For this review, take the finished solid that the model builds, in its own axes (mm). A direction names the side the tool comes from. Round coordinates to 2 decimals unless told otherwise and drop trailing zeros. Loops run counter-clockwise (first coordinate to the right, second up) from the corner with the lowest first, then second, coordinate; pieces in that order, holes last. Notation, with made-up numbers: (57.5, -3) -> (66.5, -3) arc R18 ccw to (66.5, 31) -> close; hole circle Ø5 at (12.25, 58). An arc over 180 degrees is marked (long way). Use one line per item in the form item = value. Start each with the question number.
from build123d import *

# Parameters (mm, degrees)
BOSS_EXTRUDE1_DEPTH  = 114.3
SKETCH2_W            = 6.35
SKETCH2_H            = 17.78
CUT_EXTRUDE2_DEPTH   = 99.06
SKETCH3_W            = 27.183356596
SKETCH3_H            = 83.82
CUT_EXTRUDE3_DEPTH   = 99.06
SKETCH4_W            = 27.183356596
SKETCH4_H            = 83.82
CUT_EXTRUDE4_DEPTH   = 99.06
SKETCH7_W            = 3.263536018
SKETCH7_H            = 7.713600016
CUT_EXTRUDE7_DEPTH   = 15.24
CUT_EXTRUDE8_DEPTH   = 99.06
SKETCH10_W           = 39.883356596
SKETCH10_H           = 114.3
BOSS_EXTRUDE2_DEPTH  = 7.62
CUT_EXTRUDE11_DEPTH  = 81.28
BOSS_EXTRUDE9_DEPTH  = 4.826
MIRROR9_COPY_1_DEPTH = 4.826
CUT_EXTRUDE13_DEPTH  = 19.941678176
CUT_EXTRUDE14_DEPTH  = 19.941678176
SKETCH17_W           = 27.183356538
SKETCH17_H           = 4.826
CUT_EXTRUDE15_DEPTH  = 99.06
SKETCH18_W           = 39.883356596
SKETCH18_H           = 7.62
CUT_EXTRUDE16_DEPTH  = 19.941678176
SKETCH20_W           = 27.183356538
SKETCH20_H           = 2.54
CUT_EXTRUDE19_DEPTH  = 79.118321824
FILLET1_R            = 5.08
FILLET2_R            = 2.54
SKETCH21_R           = 2.749999961
CUT_EXTRUDE20_DEPTH  = 79.118321824
SKETCH22_W           = 39.883356596
SKETCH22_H           = 5.08
BOSS_EXTRUDE10_DEPTH = 38.1
CUT_EXTRUDE21_REACH  = 169.333


with BuildPart() as part:
    # Sketch1 → Boss-Extrude1 (new body)
    with BuildSketch(Plane(origin=(0, 0, 0), x_dir=(1, 0, 0), z_dir=(0, 1, 0))):
        with BuildLine():
            Line((39.883356596, 0), (19.941678298, 34.54))
            Line((19.941678298, 34.54), (9.525, 34.54))
            Line((9.525, 34.54), (9.525, 52.32))
            Line((9.525, 52.32), (3.175, 52.32))
            Line((3.175, 52.32), (3.175, 34.54))
            Line((3.175, 34.54), (3.175, 29.28841025))
            ThreePointArc((3.175, 29.28841025), (0, -29.46), (-3.175, 29.28841025))
            Line((-3.175, 29.28841025), (-3.175, 34.54))
            Line((-3.175, 34.54), (-3.175, 52.32))
            Line((-3.175, 52.32), (-9.525, 52.32))
            Line((-9.525, 52.32), (-9.525, 34.54))
            Line((-9.525, 34.54), (-19.941678298, 34.54))
            Line((-19.941678298, 34.54), (-39.883356596, 0))
            Line((-39.883356596, 0), (-19.941678298, -34.54))
            Line((-19.941678298, -34.54), (19.941678298, -34.54))
            Line((19.941678298, -34.54), (39.883356596, 0))
        make_face()
    extrude(amount=BOSS_EXTRUDE1_DEPTH)

    # Sketch2 → Cut-Extrude2 (cut)
    with BuildSketch(Plane(origin=(0, 114.3, 0), x_dir=(1, 0, 0), z_dir=(0, 1, 0))):
        with Locations((-6.35, 43.43)):
            Rectangle(SKETCH2_W, SKETCH2_H)
        with Locations((6.35, 43.43)):
            Rectangle(SKETCH2_W, SKETCH2_H)
    extrude(amount=-CUT_EXTRUDE2_DEPTH, mode=Mode.SUBTRACT)

    # Sketch3 → Cut-Extrude3 (cut)
    with BuildSketch(Plane(origin=(-29.912517447, 0, -17.27), x_dir=(-0.49999999999999617, 0, 0.8660254037844409), z_dir=(-0.8660254037844408, 0, -0.4999999999999961))):
        with Locations((0, 57.15)):
            Rectangle(SKETCH3_W, SKETCH3_H)
    extrude(amount=-CUT_EXTRUDE3_DEPTH, mode=Mode.SUBTRACT)

    # Sketch4 → Cut-Extrude4 (cut)
    with BuildSketch(Plane(origin=(29.912517447, 0, -17.27), x_dir=(-0.500000000000004, 0, -0.8660254037844364), z_dir=(0.8660254037844365, 0, -0.500000000000004))):
        with Locations((0, 57.15)):
            Rectangle(SKETCH4_W, SKETCH4_H)
    extrude(amount=-CUT_EXTRUDE4_DEPTH, mode=Mode.SUBTRACT)

    # Sketch7 → Cut-Extrude7 (cut)
    with BuildSketch(Plane.XZ):
        with Locations((-30.838217531, 0)):
            Rectangle(SKETCH7_W, SKETCH7_H)
        with Locations((30.838217531, 0)):
            Rectangle(SKETCH7_W, SKETCH7_H)
    extrude(amount=-CUT_EXTRUDE7_DEPTH, mode=Mode.SUBTRACT)

    # Sketch8 → Cut-Extrude8 (cut)
    with BuildSketch(Plane(origin=(0, 114.3, 0), x_dir=(1, 0, 0), z_dir=(0, 1, 0))):
        Polygon((-3.175, 29.714), (3.175, 29.714), (17.155385899, 29.714), (34.310771797, 0), (17.155385899, -29.714), (-17.155385899, -29.714), (-34.310771797, 0), (-17.155385899, 29.714), align=None)
    extrude(amount=-CUT_EXTRUDE8_DEPTH, mode=Mode.SUBTRACT)

    # Sketch10 → Boss-Extrude2 (add)
    with BuildSketch(Plane.XY.offset(34.54)):
        with Locations((0, 57.15)):
            Rectangle(SKETCH10_W, SKETCH10_H)
    extrude(amount=BOSS_EXTRUDE2_DEPTH)

    # Sketch12 → Cut-Extrude11 (cut)
    with BuildSketch(Plane(origin=(-29.912517447, 0, -17.27), x_dir=(-0.4999999999999998, 0, 0.8660254037844388), z_dir=(-0.8660254037844388, 0, -0.4999999999999998))):
        Polygon((19.941678298, 114.3), (0, 114.3), (19.941678298, 94.358321702), align=None)
        Polygon((-19.941678298, 94.358321702), (0, 114.3), (-19.941678298, 114.3), align=None)
        Polygon((6.259743879, 99.06), (0, 105.319743879), (-6.259743879, 99.06), align=None)
    cut_extrude11 = extrude(amount=-CUT_EXTRUDE11_DEPTH, mode=Mode.SUBTRACT)

    # Mirror2: Cut-Extrude11 across plane
    add(cut_extrude11.mirror(Plane(origin=(0, 0, 0), x_dir=(0, 0, 1), z_dir=(1, 0, 0))), mode=Mode.SUBTRACT)

    # Sketch11 → Boss-Extrude9 (add)
    with BuildSketch(Plane(origin=(-29.912517447, 0, -17.27), x_dir=(-0.4999999999999998, 0, 0.8660254037844388), z_dir=(-0.8660254037844388, 0, -0.4999999999999998))):
        Polygon((-13.591678298, 91.728065581), (0, 105.319743879), (13.591678298, 91.728065581), (19.941678298, 94.358321702), (0, 114.3), (-19.941678298, 94.358321702), align=None)
    boss_extrude9 = extrude(amount=-BOSS_EXTRUDE9_DEPTH)

    # Mirror8: Boss-Extrude9 across plane
    add(boss_extrude9.mirror(Plane.XY))

    # Mirror9: Boss-Extrude9 across plane
    add(boss_extrude9.mirror(Plane(origin=(0, 0, 0), x_dir=(0, 0, 1), z_dir=(1, 0, 0))))

    # Mirror9 copy 1 sketch → Mirror9 copy 1 (add)
    with BuildSketch(Plane(origin=(29.912517447, 0, 17.27), x_dir=(0.4999999999999998, 0, -0.8660254037844388), z_dir=(0.8660254037844388, 0, 0.4999999999999998))):
        Polygon((-13.591678298, 91.728065581), (0, 105.319743879), (13.591678298, 91.728065581), (19.941678298, 94.358321702), (0, 114.3), (-19.941678298, 94.358321702), align=None)
    extrude(amount=-MIRROR9_COPY_1_DEPTH)

    # Sketch15 → Cut-Extrude13 (cut)
    with BuildSketch(Plane(origin=(0, 114.3, 0), x_dir=(1, 0, 0), z_dir=(0, 1, 0))):
        Polygon((-17.155385899, 29.714), (-19.941678298, 34.54), (19.941678298, 34.54), (17.155385899, 29.714), align=None)
    extrude(amount=-CUT_EXTRUDE13_DEPTH, mode=Mode.SUBTRACT)

    # Sketch16 → Cut-Extrude14 (cut)
    with BuildSketch(Plane(origin=(0, 114.3, 0), x_dir=(1, 0, 0), z_dir=(0, 1, 0))):
        Polygon((-19.941678298, -34.54), (19.941678298, -34.54), (11.5828011, -29.714), (-11.5828011, -29.714), align=None)
    extrude(amount=-CUT_EXTRUDE14_DEPTH, mode=Mode.SUBTRACT)

    # Sketch17 → Cut-Extrude15 (cut)
    with BuildSketch(Plane(origin=(0, 114.3, 0), x_dir=(1, 0, 0), z_dir=(0, 1, 0))):
        with Locations((0, -32.127)):
            Rectangle(SKETCH17_W, SKETCH17_H)
    extrude(amount=-CUT_EXTRUDE15_DEPTH, mode=Mode.SUBTRACT)

    # Sketch18 → Cut-Extrude16 (cut)
    with BuildSketch(Plane(origin=(0, 114.3, 0), x_dir=(1, 0, 0), z_dir=(0, 1, 0))):
        with Locations((0, -38.35)):
            Rectangle(SKETCH18_W, SKETCH18_H)
    extrude(amount=-CUT_EXTRUDE16_DEPTH, mode=Mode.SUBTRACT)

    # Sketch20 → Cut-Extrude19 (cut)
    with BuildSketch(Plane(origin=(0, 94.358321824, 0), x_dir=(1, 0, 0), z_dir=(0, 1, 0))):
        with Locations((0, -35.81)):
            Rectangle(SKETCH20_W, SKETCH20_H)
    extrude(amount=-CUT_EXTRUDE19_DEPTH, mode=Mode.SUBTRACT)

    # Fillet1
    fillet1_edges = [part.edges().sort_by_distance(p)[0] for p in [
        (19.941678298, 47.179160851, 34.54),
        (-39.883356596, 47.179160851, 0),
        (-19.941678298, 47.179160851, -34.54),
        (39.883356596, 47.179160851, 0),
        (-19.941678298, 47.179160851, 34.54),
        (19.941678298, 47.179160851, -34.54),
        (-9.525, 7.62, -34.54),
        (9.525, 7.62, -34.54),
    ]]
    fillet(fillet1_edges, radius=FILLET1_R)

    # Fillet2
    fillet2_edges = [part.edges().sort_by_distance(p)[0] for p in [
        (27.822798147, 114.3, 16.0635),
        (-27.822798147, 114.3, -16.0635),
        (-27.822798147, 114.3, 16.0635),
        (27.822798147, 114.3, -16.0635),
    ]]
    fillet(fillet2_edges, radius=FILLET2_R)

    # Sketch21 → Cut-Extrude20 (cut)
    with BuildSketch(Plane(origin=(9.525, 0, 0), x_dir=(0, 0, -1), z_dir=(1, 0, 0))):
        with Locations((45.97, 7.62)):
            Circle(SKETCH21_R)
    extrude(amount=-CUT_EXTRUDE20_DEPTH, mode=Mode.SUBTRACT)

    # Sketch22 → Boss-Extrude10 (add)
    with BuildSketch(Plane(origin=(0, 94.358321824, 0), x_dir=(1, 0, 0), z_dir=(0, 1, 0))):
        with Locations((0, -39.62)):
            Rectangle(SKETCH22_W, SKETCH22_H)
    extrude(amount=BOSS_EXTRUDE10_DEPTH)

    # Sketch23 → Cut-Extrude21 (cut, up to next)
    with BuildSketch(Plane.XY.offset(42.16), mode=Mode.PRIVATE) as cut_extrude21_sk1:
        with BuildLine():
            Line((2.75, 122.13), (2.75, 23.07))
            ThreePointArc((2.75, 23.07), (0, 20.32), (-2.75, 23.07))
            Line((-2.75, 23.07), (-2.75, 122.13))
            ThreePointArc((-2.75, 122.13), (0, 124.88), (2.75, 122.13))
        make_face()
    cut_extrude21_tool1 = extrude(cut_extrude21_sk1.sketch, amount=-CUT_EXTRUDE21_REACH, mode=Mode.PRIVATE) & part.part
    add(cut_extrude21_tool1.solids().sort_by_distance((0, 72.6, 42.16))[0], mode=Mode.SUBTRACT)


solid = part.part
Item 1: Take a section at C-C on y = 61. Give the number of separate pieces and of enclosed holes in the cut face, plus the area to 3 significant figures.
Item 2: Machinability: for faces 1 (the flat face through (-16, 94.358, 35)), 2 (the flat face through (-31.298, 98.429, -10.113)), 3 (the cylindrical face through (0.594, 7.513, 29.454)), which of the approach directions +Z, -Z, +X, -X, +Y, -Y give a long, thin tool a straight path to every point of the face, cutting with its end or side? Answer none if there is none.
Item 3: Wall thickness on line 1 (X direction, y = 29, z = 35.5); line 2 (Z direction, x = -10, y = 62.5); line 3 (Y direction, x = 5.5, z = -45.97): over which ranges is each line inside the solid? List them lowest first.
Item 4: Take a section at B-B on x = 0. Give the boundary of the cut face in (y, z).
Item 5: For P1, Ø2, axis at y = 90.5, z = -27, coming from the +X side; P2, Ø1.8, axis at x = -15, y = 59, coming from the -Z side; P3, Ø4, axis at y = 90, z = 40.5, coming from the -X side; P4, Ø6, axis at y = 9.5, z = 1, coming from the -X side, all flat-tipped, find the tip position at first contact; note any pin that passes through.
Item 6: Take a section at A-A on z = -45.97. Give the boundary of the cut face in (x, y) (3 decimals).
Item 7: Draft analysis for pull direction Y (two halves, no side actions). For faces 4 (the flat face through (31, 8, -3.857)), 5 (the cylindrical face through (27.808, 113.248, -16.022)), 6 (the flat face through (-2.75, 72, 40)), state which applies: +Y half, -Y half, draft (parallel to the pull), parting line (faces both ways), or undercut.
Results:
q1.separate_pieces = 6
q1.enclosed_holes = 0
q1.area = 589 mm2
q2.face_1 = +Y
q2.face_2 = none
q2.face_3 = +Y, -Y
q3.line_1 = -19.96 to -13.59, 13.59 to 19.96
q3.line_2 = -34.54 to -29.71, 37.08 to 42.16
q3.line_3 = 0 to 4.87, 10.37 to 15.24
q4.outline = (0, 29.46) -> (15.24, 29.46) -> (15.24, 37.08) -> (20.32, 37.08) -> (20.32, 42.16) -> (0, 42.16) -> close; (124.88, 37.08) -> (132.46, 37.08) -> (132.46, 42.16) -> (124.88, 42.16) -> close
q5.P1 = 21.31
q5.P2 = -34.54
q5.P3 = -19.94
q5.P4 = -39.1
q6.outline = (-9.525, 0) -> (-3.175, 0) -> (-3.175, 4.87) -> (-9.525, 4.87) -> close; (-9.525, 10.37) -> (-3.175, 10.37) -> (-3.175, 15.24) -> (-9.525, 15.24) -> close; (3.175, 0) -> (9.525, 0) -> (9.525, 4.87) -> (3.175, 4.87) -> close; (3.175, 10.37) -> (9.525, 10.37) -> (9.525, 15.24) -> (3.175, 15.24) -> close
q7.face_4 = draft
q7.face_5 = +Y half
q7.face_6 = undercut
